Verification items for this drawing (mm, ordinates from the low corner). A direction names the side the tool comes from. Round coordinates to 2 decimals unless told otherwise and drop trailing zeros. Loops run counter-clockwise (first coordinate to the right, second up) from the corner with the lowest first, then second, coordinate; pieces in that order, holes last. Notation, with made-up numbers: (5, -8) - (48, -8) arc R27 ccw to (48, 19) - close; hole circle Ø5 at (82.5, 30). An arc over 180 degrees is marked (long way). Answer in a Markdown table with one row per item. Add a question column.
(1) Thickness scan on line 1 along Y through (x, z) = (37, 15); line 2 along Y through (x, z) = (32, 20); line 3 along Z through (x, y) = (35, 65). Record the ranges inside material, lowest first.
(2) Cross-section at D-D on x = 13. Enter the section's corners in (y, z), then the cut area to 3 significant figures.
(3) Access from +Z, -Z, +X, -X, +Y, -Y to the whole of each face (thin tool, end or side, straight path). Record for the marked faces 1, 2, 3, 4 and 5.
(4) Cross-section at A-A on x = 46.5. Enter the section's corners in (y, z), then the cut area to 3 significant figures.
(5) Gauge pin test, flat ends, axial feed: pin 1 (1.5 mm diameter, centred on x = 7.5, y = 22, fed in from -Z); pin 2 (11.5 mm diameter, centred on y = 67.5, z = 27, fed in from +X); pin 3 (12 mm diameter, centred on y = 29.5, z = 20, fed in from -X); pin 4 (1.5 mm diameter, centred on x = 38, z = 25.5, fed in from -Y). Record the tip position at first contact, or that the pin passes through.
(6) Cross-section at C-C on y = 25. Enter the section's corners in (x, z), then the cut area to 3 significant figures.
(7) Cross-section at B-B on z = 5.5. Enter the section's corners in (x, y), then the cut area to 3 significant figures.
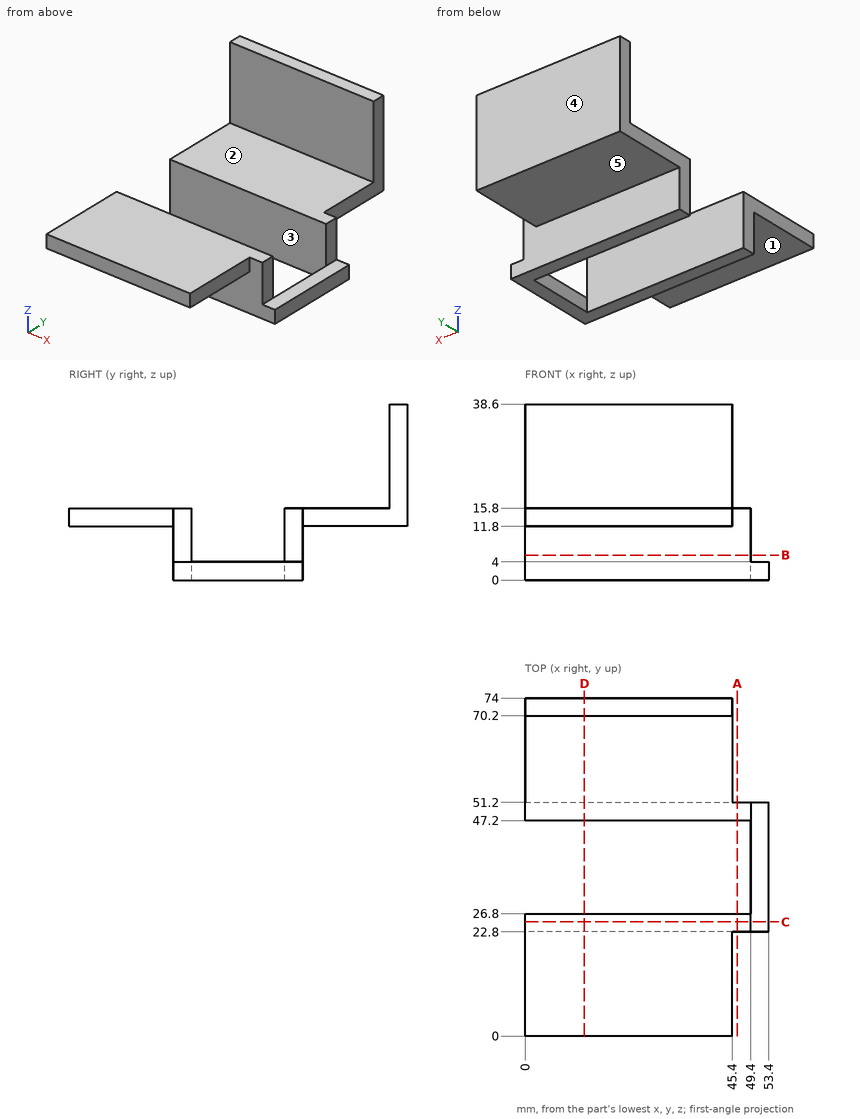
Answers:
| question | item | result |
|---|---|---|
| 1 | line 1 | y = 0 to 26.8, 47.2 to 74 |
| 1 | line 2 | y = 70.2 to 74 |
| 1 | line 3 | z = 11.8 to 15.8 |
| 2 | outline | (0, 11.8) - (22.8, 11.8) - (22.8, 0) - (26.8, 0) - (26.8, 15.8) - (0, 15.8) - close; (47.2, 0) - (51.2, 0) - (51.2, 11.8) - (74, 11.8) - (74, 38.6) - (70.2, 38.6) - (70.2, 15.8) - (47.2, 15.8) - close |
| 2 | area | 395 mm^2 |
| 3 | face 1 | -Z, +X, -X, -Y |
| 3 | face 2 | +Z, +X, -X, -Y |
| 3 | face 3 | +Z, -Z, -X |
| 3 | face 4 | +Z, -Z, +X, -X, +Y |
| 3 | face 5 | -Z, +X, -X, +Y |
| 4 | outline | (22.8, 0) - (26.8, 0) - (26.8, 15.8) - (22.8, 15.8) - close; (47.2, 0) - (51.2, 0) - (51.2, 15.8) - (47.2, 15.8) - close |
| 4 | area | 126 mm^2 |
| 5 | pin 1 | stops at z = 11.8 |
| 5 | pin 2 | stops at x = 45.4 |
| 5 | pin 3 | stops at x = 0 |
| 5 | pin 4 | stops at y = 70.2 |
| 6 | outline | (0, 0) - (53.4, 0) - (53.4, 4) - (49.4, 4) - (49.4, 15.8) - (0, 15.8) - close |
| 6 | area | 797 mm^2 |
| 7 | outline | (0, 22.8) - (49.4, 22.8) - (49.4, 26.8) - (0, 26.8) - close; (0, 47.2) - (49.4, 47.2) - (49.4, 51.2) - (0, 51.2) - close |
| 7 | area | 395 mm^2 |
